```python
from build123d import *

# Parameters (mm, degrees)
SKETCH1_W           = 16.764
SKETCH1_H           = 16.764
BOSS_EXTRUDE1_DEPTH = 13.97
SKETCH2_R           = 3.175
BOSS_EXTRUDE2_DEPTH = 2.54
SKETCH3_R           = 3.175
BOSS_EXTRUDE3_DEPTH = 2.54


with BuildPart() as part:
    # Sketch1 → Boss-Extrude1 (new body)
    with BuildSketch(Plane(origin=(0, 0, 0), x_dir=(1, 0, 0), z_dir=(0, 1, 0))):
        Rectangle(SKETCH1_W, SKETCH1_H)
    extrude(amount=BOSS_EXTRUDE1_DEPTH)

    # Sketch2 → Boss-Extrude2 (add)
    with BuildSketch(Plane.XY.offset(8.382)):
        with Locations((0, 6.985)):
            Circle(SKETCH2_R)
    boss_extrude2 = extrude(amount=BOSS_EXTRUDE2_DEPTH)

    # Mirror1: Boss-Extrude2 across plane
    add(boss_extrude2.mirror(Plane.XY))

    # Sketch3 → Boss-Extrude3 (add)
    with BuildSketch(Plane(origin=(8.382, 0, 0), x_dir=(0, 0, -1), z_dir=(1, 0, 0))):
        with Locations((0, 6.985)):
            Circle(SKETCH3_R)
    boss_extrude3 = extrude(amount=BOSS_EXTRUDE3_DEPTH)

    # Mirror2: Boss-Extrude3 across plane
    add(boss_extrude3.mirror(Plane(origin=(0, 0, 0), x_dir=(0, 0, 1), z_dir=(1, 0, 0))))


solid = part.part
```
Geometry check sheet. Reference: the model listing, model coordinates, mm. A direction names the side the tool comes from. Coordinates: 2 decimals unless noted, no trailing zeros. Write each loop counter-clockwise with the first axis right and the second up, starting at its lowest first coordinate (ties: lowest second). Pieces come first, ordered by that corner, then holes. Notation, with made-up numbers: M 89.25,-13 L 129.25,-13 A29 cw 129.25,26 Z; hole C -14,88.5 d1. An arc over 180 degrees is marked long. One line per item, written item: value. Start each with the question number.
(1) Scan lines: line 1 along X through (y, z) = (2.75, -2.25); line 2 along Z through (x, y) = (-8.5, 4.5). Record each from-to range of solid material in increasing order. Write a range as [from, to].
(2) Sectioned sample at A-A, the plane z = 0. Enter the section's corners in (x, y), and give its area (3 significant figures).
(3) Tool access check on faces 1 (the face through (-2.52, 5.053, -9.634)), 2 (the face through (-9.634, 5.053, 2.52)), 3 (the face through (9.634, 5.053, 2.52)), 4 (the face through (-2.52, 5.053, 9.634)). Record the directions out of +Z, -Z, +X, -X, +Y, -Y that give a thin tool (end or side, any length) a straight path to the whole face; none if there is none.
(4) Sectioned sample at D-D, the plane y = 1.5. Enter the section's corners in (x, z).
(5) Sectioned sample at C-C, the plane y = 8.75. Enter the section's corners in (x, z).
(6) Depth check by flat-ended pin: pin 1 (3 mm diameter, centred on x = -7, y = 5.5, fed in from -Z); pin 2 (2 mm diameter, centred on y = 11.5, z = -0.5, fed in from -X). Enter the tip coordinate at first touch or a pass-through.
(7) Sectioned sample at B-B, the plane x = 0. Enter the section's corners in (y, z).
Filled sheet:
1. line 1: [-8.38, 8.38]
1. line 2: [-1.98, 1.98]
2. outline: M -10.92,3.81 L -8.38,3.81 L -8.38,0 L 8.38,0 L 8.38,3.81 L 10.92,3.81 L 10.92,10.16 L 8.38,10.16 L 8.38,13.97 L -8.38,13.97 L -8.38,10.16 L -10.92,10.16 Z
2. area: 266 mm²
3. face 1: -Z
3. face 2: -X
3. face 3: +X
3. face 4: +Z
4. outline: M -8.38,-8.38 L 8.38,-8.38 L 8.38,8.38 L -8.38,8.38 Z
5. outline: M -10.92,-2.64 L -8.38,-2.64 L -8.38,-8.38 L -2.64,-8.38 L -2.64,-10.92 L 2.64,-10.92 L 2.64,-8.38 L 8.38,-8.38 L 8.38,-2.64 L 10.92,-2.64 L 10.92,2.64 L 8.38,2.64 L 8.38,8.38 L 2.64,8.38 L 2.64,10.92 L -2.64,10.92 L -2.64,8.38 L -8.38,8.38 L -8.38,2.64 L -10.92,2.64 Z
6. pin 1: z = -8.38
6. pin 2: x = -8.38
7. outline: M 0,-8.38 L 3.81,-8.38 L 3.81,-10.92 L 10.16,-10.92 L 10.16,-8.38 L 13.97,-8.38 L 13.97,8.38 L 10.16,8.38 L 10.16,10.92 L 3.81,10.92 L 3.81,8.38 L 0,8.38 Z
